```python
from build123d import *

# Parameters (mm, degrees)
SKETCH1_W                                 = 12.7
SKETCH1_H                                 = 148.079451403
BOSS_EXTRUDE1_DEPTH                       = 342.9
F_15_64_0_23438_DIAMETER_HOLE1_D          = 5.953252
F_15_64_0_23438_DIAMETER_HOLE1_DEPTH      = 12.7
F_15_64_0_23438_DIAMETER_HOLE1_TIP        = 1.788537341
F_15_64_0_23438_DIAMETER_HOLE3_D          = 5.953252
F_15_64_0_23438_DIAMETER_HOLE3_DEPTH      = 19.05
F_15_64_0_23438_DIAMETER_HOLE3_TIP        = 1.788537341
F_5_64_0_07813_DIAMETER_HOLE1_D           = 1.984502
F_5_64_0_07813_DIAMETER_HOLE1_DEPTH       = 38.1
F_5_64_0_07813_DIAMETER_HOLE1_CSINK_D     = 10.16
F_5_64_0_07813_DIAMETER_HOLE1_CSINK_ANGLE = 82
F_5_64_0_07813_DIAMETER_HOLE1_TIP         = 0.59620455
F_5_64_0_07813_DIAMETER_HOLE2_D           = 1.984502
F_5_64_0_07813_DIAMETER_HOLE2_DEPTH       = 38.1
F_5_64_0_07813_DIAMETER_HOLE2_CSINK_D     = 10.16
F_5_64_0_07813_DIAMETER_HOLE2_CSINK_ANGLE = 82
F_5_64_0_07813_DIAMETER_HOLE2_TIP         = 0.59620455
F_8_CLEARANCE_HOLE1_D                     = 4.9149
F_8_CLEARANCE_HOLE1_DEPTH                 = 12.7
CUT_EXTRUDE1_REACH                        = 14.7
SKETCH14_R                                = 51.814725701
CUT_EXTRUDE2_REACH                        = 14.7


with BuildPart() as part:
    # Sketch1 → Boss-Extrude1 (new body)
    with BuildSketch(Plane.XY):
        with Locations((-445.23025, -77.214725702)):
            Rectangle(SKETCH1_W, SKETCH1_H)
    extrude(amount=BOSS_EXTRUDE1_DEPTH)

    # 15/64 (0.23438) Diameter Hole1
    with Locations(Plane(origin=(-183.67375, 1933.375856936, -6.35), x_dir=(1, 0, 0), z_dir=(0, 0, -1))):
        with Locations((-261.5565, 1973.570719787), (-261.5565, 2010.590582637), (-261.5565, 2047.610445488), (-97.5233, 2112.481693679), (-97.5233, 2147.688356936), (-43.36415, 2120.065856936), (1.27, 2120.065856936), (45.90415, 2120.065856936), (100.0633, 2147.688356936), (100.0633, 2112.481693679), (264.0965, 2047.610445488), (264.0965, 1973.570719787)):
            Hole(F_15_64_0_23438_DIAMETER_HOLE1_D / 2, depth=F_15_64_0_23438_DIAMETER_HOLE1_DEPTH)
            with Locations((0, 0, -(F_15_64_0_23438_DIAMETER_HOLE1_DEPTH + F_15_64_0_23438_DIAMETER_HOLE1_TIP / 2))):  # 118° drill point
                Cone(0, F_15_64_0_23438_DIAMETER_HOLE1_D / 2, F_15_64_0_23438_DIAMETER_HOLE1_TIP, mode=Mode.SUBTRACT)

    # 15/64 (0.23438) Diameter Hole3
    with Locations(Plane(origin=(-182.40375, 1936.853954382, -6.35), x_dir=(1, 0, 0), z_dir=(0, 0, -1))):
        with Locations((-262.8265, 2051.088542934), (-262.8265, 2014.068680083), (-262.8265, 1977.048817232), (-98.7933, 2115.959791125), (-98.7933, 2151.166454382)):
            Hole(F_15_64_0_23438_DIAMETER_HOLE3_D / 2, depth=F_15_64_0_23438_DIAMETER_HOLE3_DEPTH)
            with Locations((0, 0, -(F_15_64_0_23438_DIAMETER_HOLE3_DEPTH + F_15_64_0_23438_DIAMETER_HOLE3_TIP / 2))):  # 118° drill point
                Cone(0, F_15_64_0_23438_DIAMETER_HOLE3_D / 2, F_15_64_0_23438_DIAMETER_HOLE3_TIP, mode=Mode.SUBTRACT)

    # 5/64 (0.07813) Diameter Hole1
    with Locations(Plane(origin=(-182.40375, 15.875, 6471.459863233), x_dir=(1, 0, 0), z_dir=(0, 1, 0))):
        with Locations((-262.8265, 6157.452363233), (-98.7933, 6157.452363233), (-262.8265, 6233.652363233), (-98.7933, 6233.652363233), (-262.8265, 6309.852363233), (-98.7933, 6309.852363233), (-267.97, 6119.034863233), (-115.57, 6119.034863233), (-1.27, 6119.034863233), (113.03, 6119.034863233), (265.43, 6119.034863233), (96.2533, 6309.852363233), (260.2865, 6309.852363233), (96.2533, 6233.652363233), (260.2865, 6233.652363233), (96.2533, 6157.452363233), (260.2865, 6157.452363233)):
            CounterSinkHole(F_5_64_0_07813_DIAMETER_HOLE1_D / 2, F_5_64_0_07813_DIAMETER_HOLE1_CSINK_D / 2, depth=F_5_64_0_07813_DIAMETER_HOLE1_DEPTH, counter_sink_angle=F_5_64_0_07813_DIAMETER_HOLE1_CSINK_ANGLE)
            with Locations((0, 0, -(F_5_64_0_07813_DIAMETER_HOLE1_DEPTH + F_5_64_0_07813_DIAMETER_HOLE1_TIP / 2))):  # 118° drill point
                Cone(0, F_5_64_0_07813_DIAMETER_HOLE1_D / 2, F_5_64_0_07813_DIAMETER_HOLE1_TIP, mode=Mode.SUBTRACT)

    # 5/64 (0.07813) Diameter Hole2
    with Locations(Plane(origin=(-182.40375, 1936.853954382, 361.95), x_dir=(-1, 0, 0), z_dir=(0, 0, 1))):
        with Locations((-263.392416364, 1965.434682144), (262.8265, 1964.708862949), (262.8265, 2063.428497217), (98.7933, 2131.851871048), (98.7933, 1978.393537715), (53.56098, 2123.543954382), (-53.56098, 2123.543954382), (-99.322089753, 1978.666800322), (-98.898757225, 2132.124549748), (-263.120086856, 2064.153940785)):
            CounterSinkHole(F_5_64_0_07813_DIAMETER_HOLE2_D / 2, F_5_64_0_07813_DIAMETER_HOLE2_CSINK_D / 2, depth=F_5_64_0_07813_DIAMETER_HOLE2_DEPTH, counter_sink_angle=F_5_64_0_07813_DIAMETER_HOLE2_CSINK_ANGLE)
            with Locations((0, 0, -(F_5_64_0_07813_DIAMETER_HOLE2_DEPTH + F_5_64_0_07813_DIAMETER_HOLE2_TIP / 2))):  # 118° drill point
                Cone(0, F_5_64_0_07813_DIAMETER_HOLE2_D / 2, F_5_64_0_07813_DIAMETER_HOLE2_TIP, mode=Mode.SUBTRACT)

    # #8 Clearance Hole1
    with Locations(Plane.ZY.offset(451.58025)):
        with Locations((88.9, -27.7495), (35.8275, -27.7495), (38.1, -128.5875)):
            Hole(F_8_CLEARANCE_HOLE1_D / 2, depth=F_8_CLEARANCE_HOLE1_DEPTH)

    # Sketch14 → Cut-Extrude1 (cut, up to next)
    with BuildSketch(Plane.ZY.offset(451.58025), mode=Mode.PRIVATE) as cut_extrude1_sk1:
        with Locations((250.825, -77.214725701)):
            Circle(SKETCH14_R)
    cut_extrude1_tool1 = extrude(cut_extrude1_sk1.sketch, amount=-CUT_EXTRUDE1_REACH, mode=Mode.PRIVATE) & part.part
    add(cut_extrude1_tool1.solids().sort_by_distance((-451.58025, -77.214726, 250.825))[0], mode=Mode.SUBTRACT)

    # Sketch15 → Cut-Extrude2 (cut, up to next)
    with BuildSketch(Plane.ZY.offset(451.58025), mode=Mode.PRIVATE) as cut_extrude2_sk1:
        with BuildLine():
            Line((92.8625, -60.322451403), (57.9375, -60.322451403))
            ThreePointArc((57.9375, -60.322451403), (51.5875, -53.972451403), (57.9375, -47.622451403))
            Line((57.9375, -47.622451403), (92.8625, -47.622451403))
            ThreePointArc((92.8625, -47.622451403), (99.2125, -53.972451403), (92.8625, -60.322451403))
        make_face()
    cut_extrude2_tool1 = extrude(cut_extrude2_sk1.sketch, amount=-CUT_EXTRUDE2_REACH, mode=Mode.PRIVATE) & part.part
    add(cut_extrude2_tool1.solids().sort_by_distance((-451.58025, -53.972451, 75.4))[0], mode=Mode.SUBTRACT)


solid = part.part
```
Could you check a few things on this model? Use its own coordinates, in mm. A direction names the side the tool comes from. Coordinates: 2 decimals unless noted, no trailing zeros. Write each loop counter-clockwise with the first axis right and the second up, starting at its lowest first coordinate (ties: lowest second). Pieces come first, ordered by that corner, then holes. Notation, with made-up numbers: (36, 54.25) - (65, 54.25) arc R15 ccw to (65, 64.25) - close; hole circle Ø9 at (72.5, 4.25). An arc over 180 degrees is marked (long way). Use a Markdown table: item, result.
Q1. Thinking about a two-plate mould opening in Y: for faces 1 (the conical face through (-445.34, -113.73, 14.18)), 2 (the flat face through (-438.88, -78, 169)), 3 (the flat face through (-445, -3.175, 169)), 4 (the cylindrical face through (-445.32, -74.94, 199.06)), which applies, +Y half, -Y half, draft (parallel to the pull), parting line (faces both ways), or undercut?
Geometry check:
| item | result |
|---|---|
| face 1 | undercut |
| face 2 | draft |
| face 3 | +Y half |
| face 4 | undercut |
Q2. Imagine slicing it at A-A (z = 75). List the corners of the cut face in (x, y) for me (3 decimals).
Geometry check:
| item | result |
|---|---|
| outline | (-451.58, -151.254) - (-438.88, -151.254) - (-438.88, -60.322) - (-451.58, -60.322) - close; (-451.58, -47.622) - (-438.88, -47.622) - (-438.88, -3.175) - (-451.58, -3.175) - close |
Q3. Please list where these lines run through material, in increasing order: L1, parallel to Z at x = -449.25, y = -64; L2, parallel to Z at x = -445.25, y = -97; L3, parallel to Y at x = -443.75, z = 273.5 (3 decimals).
Geometry check:
| item | result |
|---|---|
| L1 | z = 0 to 200.72, 300.93 to 342.9 |
| L2 | z = 0 to 202.94, 298.71 to 342.9 |
| L3 | y = -151.254 to -123.805, -30.625 to -3.175 |
Q4. Imagine slicing it at B-B (y = -91). List the corners of the cut face in (x, z) for me, and give its area (3 significant figures).
Geometry check:
| item | result |
|---|---|
| outline | (-451.58, 0) - (-438.88, 0) - (-438.88, 200.88) - (-451.58, 200.88) - close; (-451.58, 300.77) - (-438.88, 300.77) - (-438.88, 342.9) - (-451.58, 342.9) - close |
| area | 3,090 mm2 |
Q5. Which directions (+Z, -Z, +X, -X, +Y, -Y) give clear straight access to the entire face, cutting with the end or side of a thin tool? Please do faces 5 (the cylindrical face through (-448, -39.1, 6.4)), 6 (the flat face through (-450, -76, 0)), 7 (the cylindrical face through (-445.32, -53.83, 99.21)).
Geometry check:
| item | result |
|---|---|
| face 5 | -Z |
| face 6 | -Z, +X, -X, +Y, -Y |
| face 7 | +X, -X |
